from build123d import *

# Parameters (mm, degrees)
SKETCH1_R               = 60
SKETCH1_R_2             = 1.5
BOSS_EXTRUDE1_DEPTH     = 5
SKETCH2_W               = 5
SKETCH2_H               = 75
BOSS_EXTRUDE2_DEPTH     = 50
SKETCH3_R               = 1.5
SKETCH3_R_2             = 12.5
CUT_EXTRUDE1_DEPTH      = 122.063000128
CUT_EXTRUDE4_DEPTH      = 101.031245119
CUT_EXTRUDE4_DEPTH_BACK = 53
SKETCH5_R               = 2.24506403
SKETCH6_R               = 1.5
SKETCH6_R_2             = 12.5
CUT_EXTRUDE5_DEPTH      = 5
SKETCH7_R               = 2.5
BOSS_EXTRUDE4_DEPTH     = 5
BODY_MOVE_COPY1_ANGLE   = 180


with BuildPart() as part:
    # Sketch1 → Boss-Extrude1 (new body)
    with BuildSketch(Plane.XY):
        Circle(SKETCH1_R)
        Circle(SKETCH1_R_2, mode=Mode.SUBTRACT)
    extrude(amount=BOSS_EXTRUDE1_DEPTH)

    # Sketch2 → Boss-Extrude2 (add)
    with BuildSketch(Plane(origin=(0, 0, 0), x_dir=(-1, 0, 0), z_dir=(0, 0, -1))):
        with Locations((-35, 0)):
            Rectangle(SKETCH2_W, SKETCH2_H)
        with Locations((35, 0)):
            Rectangle(SKETCH2_W, SKETCH2_H)
        Rectangle(SKETCH2_W, SKETCH2_H)
    extrude(amount=BOSS_EXTRUDE2_DEPTH)

    # Sketch3 → Cut-Extrude1 (cut, through all)
    with BuildSketch(Plane.ZY.offset(-32.5)):
        with Locations(Location((-40.5, 3, 0), (0, 0, 270))):
            Circle(SKETCH3_R)
        with Locations(Location((-9.5, 3, 0), (0, 0, 270))):
            Circle(SKETCH3_R)
        with Locations(Location((-9.5, -28, 0), (0, 0, 270))):
            Circle(SKETCH3_R)
        with Locations(Location((-40.5, -28, 0), (0, 0, 270))):
            Circle(SKETCH3_R)
        with Locations(Location((-25, -12.5, 0), (0, 0, 270))):
            Circle(SKETCH3_R_2)
    extrude(amount=-CUT_EXTRUDE1_DEPTH, mode=Mode.SUBTRACT)

    # Sketch5 → Cut-Extrude4 (cut, two sides: drawn at the far end of the back side and taken through both)
    with BuildSketch(Plane.ZY.offset(2.5).offset(-CUT_EXTRUDE4_DEPTH_BACK)):
        with Locations(Location((-25, 12.5, 0), (0, 0, 180))):
            Circle(SKETCH5_R)
    extrude(amount=CUT_EXTRUDE4_DEPTH + CUT_EXTRUDE4_DEPTH_BACK, mode=Mode.SUBTRACT)

    # Sketch6 → Cut-Extrude5 (cut)
    with BuildSketch(Plane.ZY.offset(37.5)):
        with Locations(Location((-40.5, 3, 0), (0, 0, 270))):
            Circle(SKETCH6_R)
        with Locations(Location((-9.5, 3, 0), (0, 0, 270))):
            Circle(SKETCH6_R)
        with Locations(Location((-9.5, -28, 0), (0, 0, 270))):
            Circle(SKETCH6_R)
        with Locations(Location((-40.5, -28, 0), (0, 0, 270))):
            Circle(SKETCH6_R)
        with Locations(Location((-25, -12.5, 0), (0, 0, 270))):
            Circle(SKETCH6_R_2)
    extrude(amount=-CUT_EXTRUDE5_DEPTH, mode=Mode.SUBTRACT)

    # Sketch7 → Boss-Extrude4 (add)
    with BuildSketch(Plane.ZY.offset(37.5)):
        with BuildLine():
            Line((-50, 37.5), (-64.138546099, 30.534707883))
            ThreePointArc((-64.138546099, 30.534707883), (-68.91560159, 22.940582469), (-64.290723579, 15.252832254))
            Line((-64.290723579, 15.252832254), (-50, 7.855339059))
            Line((-50, 7.855339059), (-50, 37.5))
        make_face()
        with Locations(Location((-60.355339059, 22.855339059, 0), (0, 0, 270))):
            Circle(SKETCH7_R, mode=Mode.SUBTRACT)
    extrude(amount=-BOSS_EXTRUDE4_DEPTH)


with BuildPart() as part_1:
    # Body-Move/Copy1: moved
    add(part.part.rotate(Axis((0, 0, -31.958013004), (1, 0, 0)), BODY_MOVE_COPY1_ANGLE))


with BuildPart() as part_2:
    # Body-Move/Copy2: moved
    add(part_1.part.moved(Location((0, 0, 68.91602601))))


solid = part_2.part
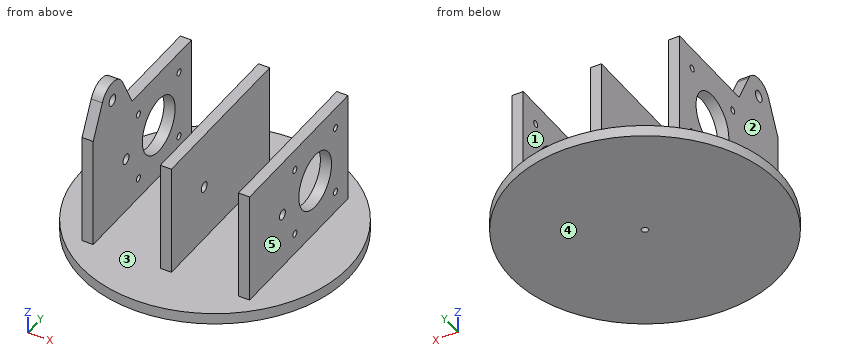
Can you work these out from the model? Positions are in its coordinate system, mm. Face numbers are marked on the shaded views. A direction names the side the tool comes from. Round coordinates to 2 decimals unless told otherwise and drop trailing zeros. Write each loop counter-clockwise with the first axis right and the second up, starting at its lowest first coordinate (ties: lowest second). Pieces come first, ordered by that corner, then holes. Notation, with made-up numbers: M 28,32 L 47,32 A7 cw 47,39 Z; hole C -24,56 d4. An arc over 180 degrees is marked long. Use CSV: the item, a comma, the result in double quotes.
(1) I need wall thicknesses on line 1 along Z through (x, y) = (-34.8, 28); line 2 along X through (y, z) = (-3.5, 17); line 3 along Z through (x, y) = (-32, -7.5). Which ranges of each line are inside material? Lowest first, please.
Check values:
line 1,"0 to 13, 16 to 44, 47 to 55"
line 2,"-37.5 to -32.5, -2.5 to 2.5, 32.5 to 37.5"
line 3,"0 to 5"
(2) Imagine slicing it at B-B (z = 14.5). Write out the boundary of the cut face in (x, y), plus the area to 4 significant figures.
Check values:
outline,"M -37.5,-37.5 L -32.5,-37.5 L -32.5,-4.5 L -37.5,-4.5 Z; M -37.5,-1.5 L -32.5,-1.5 L -32.5,26.5 L -37.5,26.5 Z; M -37.5,29.5 L -32.5,29.5 L -32.5,37.5 L -37.5,37.5 Z; M -2.5,-37.5 L 2.5,-37.5 L 2.5,37.5 L -2.5,37.5 Z; M 32.5,-37.5 L 37.5,-37.5 L 37.5,-4.5 L 32.5,-4.5 Z; M 32.5,-1.5 L 37.5,-1.5 L 37.5,26.5 L 32.5,26.5 Z; M 32.5,29.5 L 37.5,29.5 L 37.5,37.5 L 32.5,37.5 Z"
area,"1,065 mm^2"
(3) Imagine slicing it at A-A (z = 22.5). Write out the boundary of the cut face in (x, y).
Check values:
outline,"M -37.5,-37.5 L -32.5,-37.5 L -32.5,2.5 L -37.5,2.5 Z; M -37.5,22.5 L -32.5,22.5 L -32.5,37.5 L -37.5,37.5 Z; M -2.5,-37.5 L 2.5,-37.5 L 2.5,37.5 L -2.5,37.5 Z; M 32.5,-37.5 L 37.5,-37.5 L 37.5,2.5 L 32.5,2.5 Z; M 32.5,22.5 L 37.5,22.5 L 37.5,37.5 L 32.5,37.5 Z"
(4) Imagine slicing it at D-D (y = 12.5). Write out the boundary of the cut face in (x, z).
Check values:
outline,"M -58.68,0 L 58.68,0 L 58.68,5 L 37.5,5 L 37.5,17.5 L 32.5,17.5 L 32.5,5 L 2.5,5 L 2.5,55 L -2.5,55 L -2.5,5 L -32.5,5 L -32.5,17.5 L -37.5,17.5 L -37.5,5 L -58.68,5 Z; M -37.5,42.5 L -32.5,42.5 L -32.5,55 L -37.5,55 Z; M 32.5,42.5 L 37.5,42.5 L 37.5,55 L 32.5,55 Z"
(5) On a 3-axis mill with a long thin cutter (end or side, diameter ignored), from which of +Z, -Z, +X, -X, +Y, -Y can I reach the whole of each face in a straight line? I mean the marked faces 1 and 2. Say none if no direction works.
Check values:
face 1,"+Z, +Y, -Y"
face 2,"+Z, -X, +Y, -Y"
(6) We'd pull the mould along X, two halves only. Please class the marked faces 3, 4 and 5: +X half, -X half, draft (parallel to the pull), parting line (faces both ways), or undercut.
Check values:
face 3,"undercut"
face 4,"draft"
face 5,"+X half"
(7) I'm going to push flat-ended pins straight in: pin 1 (2.5 mm diameter, centred on x = 0, y = 0, fed in from +Z); pin 2 (3.5 mm diameter, centred on y = 28, z = 14.5, fed in from -X); pin 3 (12 mm diameter, centred on x = -7, z = 54, fed in from +Y). Where does each tip first touch, or does it pass through?
Check values:
pin 1,"z = 55"
pin 2,"x = -37.5"
pin 3,"y = 37.5"
(8) Imagine slicing it at C-C (x = 0). Write out the boundary of the cut face in (y, z).
Check values:
outline,"M -60,0 L -1.5,0 L -1.5,5 L 1.5,5 L 1.5,0 L 60,0 L 60,5 L 37.5,5 L 37.5,55 L -37.5,55 L -37.5,5 L -60,5 Z; hole C -12.5,30 d4.49"
